Geometry: final body of the model. Coordinates: model frame, mm. A direction names the side the tool comes from. Coordinates: 2 decimals unless noted, no trailing zeros. Write each loop counter-clockwise with the first axis right and the second up, starting at its lowest first coordinate (ties: lowest second). Pieces come first, ordered by that corner, then holes. Notation, with made-up numbers: (13.5, 66) - (53.5, 66) arc R17 ccw to (53.5, 93) - close; hole circle Ø9 at (28.5, -0.75). An arc over 180 degrees is marked (long way). Put each result on its own line as item: value.
```python
from build123d import *

# Parameters (mm, degrees)
SKETCH2_W           = 500
SKETCH2_H           = 228.2
BOSS_EXTRUDE1_DEPTH = 10
SKETCH3_W           = 200
SKETCH3_H           = 30
CUT_EXTRUDE1_DEPTH  = 10
FILLET1_R           = 4
CUT_EXTRUDE2_REACH  = 502


with BuildPart() as part:
    # Sketch2 → Boss-Extrude1 (new body)
    with BuildSketch(Plane(origin=(0, 0, 0), x_dir=(1, 0, 0), z_dir=(0, 1, 0))):
        Rectangle(SKETCH2_W, SKETCH2_H)
    extrude(amount=BOSS_EXTRUDE1_DEPTH)

    # Sketch3 → Cut-Extrude1 (cut)
    with BuildSketch(Plane(origin=(0, 10, 0), x_dir=(1, 0, 0), z_dir=(0, 1, 0))):
        with Locations((0, 79.1)):
            Rectangle(SKETCH3_W, SKETCH3_H)
    extrude(amount=-CUT_EXTRUDE1_DEPTH, mode=Mode.SUBTRACT)

    # Fillet1
    fillet1_edges = [part.edges().sort_by_distance(p)[0] for p in [
        (100, 5, -94.1),
        (100, 5, -64.1),
        (-100, 5, -64.1),
        (-100, 5, -94.1),
    ]]
    fillet(fillet1_edges, radius=FILLET1_R)

    # Sketch4 → Cut-Extrude2 (cut, up to next)
    with BuildSketch(Plane(origin=(250, 0, 0), x_dir=(0, 0, -1), z_dir=(1, 0, 0)), mode=Mode.PRIVATE) as cut_extrude2_sk1:
        Polygon((114.1, 0), (111.791318089, 10), (114.1, 10), align=None)
    cut_extrude2_tool1 = extrude(cut_extrude2_sk1.sketch, amount=-CUT_EXTRUDE2_REACH, mode=Mode.PRIVATE) & part.part
    add(cut_extrude2_tool1.solids().sort_by_distance((250, 6.666667, -113.330439))[0], mode=Mode.SUBTRACT)
    # Sketch4 → Cut-Extrude2 (cut, up to next)
    with BuildSketch(Plane(origin=(250, 0, 0), x_dir=(0, 0, -1), z_dir=(1, 0, 0)), mode=Mode.PRIVATE) as cut_extrude2_sk2:
        Polygon((-114.1, 0), (-114.1, 10), (-111.791318089, 0), align=None)
    cut_extrude2_tool2 = extrude(cut_extrude2_sk2.sketch, amount=-CUT_EXTRUDE2_REACH, mode=Mode.PRIVATE) & part.part
    add(cut_extrude2_tool2.solids().sort_by_distance((250, 3.333333, 113.330439))[0], mode=Mode.SUBTRACT)


solid = part.part
```
1. Set-up query: faces 1 (the flat face through (-3, 0, -3)), 2 (the flat face through (-100, 5, -79)). Return all of +Z, -Z, +X, -X, +Y, -Y with unobstructed straight access to the full face (end or side cutting, diameter ignored); none if empty.
Answer below:
face 1: +Z, -Z, +X, -X, -Y
face 2: +Y, -Y
2. Section query B-B (z = -82.5). Return loops of the section in (x, y).
Answer below:
outline: (-250, 0) - (-100, 0) - (-100, 10) - (-250, 10) - close; (100, 0) - (250, 0) - (250, 10) - (100, 10) - close
3. Pin query (flat end, axial travel): pin 1 Ø5 at (x, y) = (176, 3) entering from +Z; pin 2 Ø3 at (x, y) = (-102.5, 4.5) entering from +Z; pin 3 Ø1.5 at (x, y) = (72.5, 6) entering from -Z; pin 4 Ø1.5 at (x, z) = (19.5, 0.5) entering from -Y. Return the tip coordinate at first contact, or that it passes through.
Answer below:
pin 1: stops at z = 113.06
pin 2: stops at z = 113.18
pin 3: stops at z = -112.89
pin 4: stops at y = 0
4. Ray query, probe 1 along Z at (x, y) = (-61, 8.5); probe 2 along Z at (x, y) = (0, 2.75); probe 3 along Z at (x, y) = (188, 8.75). Return the intervals inside material, ascending. Write a range as from..to.
Answer below:
probe 1: z = -112.14..-94.1, -64.1..113.75
probe 2: z = -113.47..-94.1, -64.1..112.43
probe 3: z = -112.08..113.81
5. Mould query, pull axis X, two halves, no side actions, for faces 3 (the flat face through (100, 5, -79)), 4 (the flat face through (250, 5, 2)), 5 (the flat face through (-1, 5, -64.1)), 6 (the flat face through (3.5, 5.07, 112.96)). Classes: +X half, -X half, draft (parallel to the pull), parting line (faces both ways), or undercut.
Answer below:
face 3: undercut
face 4: +X half
face 5: undercut
face 6: draft
6. Section query C-C (y = 6). Return loops of the section in (x, z).
Answer below:
outline: (-250, -112.71) - (250, -112.71) - (250, 113.18) - (-250, 113.18) - close; hole (-100, -90.1) arc R4 ccw to (-96, -94.1) - (96, -94.1) arc R4 ccw to (100, -90.1) - (100, -68.1) arc R4 ccw to (96, -64.1) - (-96, -64.1) arc R4 ccw to (-100, -68.1) - close
7. Section query A-A (x = 2). Return loops of the section in (y, z), then the cut area to 3 significant figures.
Answer below:
outline: (0, -114.1) - (10, -111.79) - (10, -94.1) - (0, -94.1) - close; (0, -64.1) - (10, -64.1) - (10, 114.1) - (0, 111.79) - close
area: 1,960 mm²
